Can you work these out from the drawing? Everything is in mm from the part's minimum corner. A direction names the side the tool comes from. Coordinates: 2 decimals unless noted, no trailing zeros. Write each loop counter-clockwise with the first axis right and the second up, starting at its lowest first coordinate (ties: lowest second). Pieces come first, ordered by that corner, then holes. Notation, with made-up numbers: (-7, 39.25) -> (14, 39.25) arc R29 cw to (14, 64.25) -> close; hole circle Ø2 at (82.5, 25). An arc over 180 degrees is marked (long way). Use a Markdown table: item, result. Add a question column.
Item 1: On a 3-axis mill with a long thin cutter (end or side, diameter ignored), from which of +Z, -Z, +X, -X, +Y, -Y can I reach the whole of each face in a straight line? I mean the marked faces 4, 5, 6 and 7. Say none if no direction works.
Item 2: If we mould it in two halves opening along Z, with no side actions, what happens to the marked faces 1, 2 and 3? For each: pulls with the +Z half, pulls with the -Z half, needs draft (parallel to the pull), parting line crosses it, or undercut.
Item 3: Imagine slicing it at A-A, the plane y = 1.5. Write out the boundary of the cut face in (x, z).
Item 4: Will these pins go through, and if not, where does the flat tip stop? pin 1 Ø3.5 at (y, z) = (12, 37.5) entering from +X; pin 2 Ø1.5 at (x, z) = (99.5, 46.5) entering from +Y.
Item 5: Imagine slicing it at B-B, the plane z = 23.5. Write out the boundary of the cut face in (x, y), and give its area (3 significant figures).
Item 6: If I drill on line 1 along X through (y, z) = (2.5, 27.5); line 2 along X through (y, z) = (2.25, 60); line 3 along Y through (x, z) = (103.5, 53.5), over which ranges is the centre line in solid material (lowest first)? Write a range as from..to.
Item 7: Imagine slicing it at C-C, the plane x = 74.5. Write out the boundary of the cut face in (y, z), and give its area (3 significant figures).
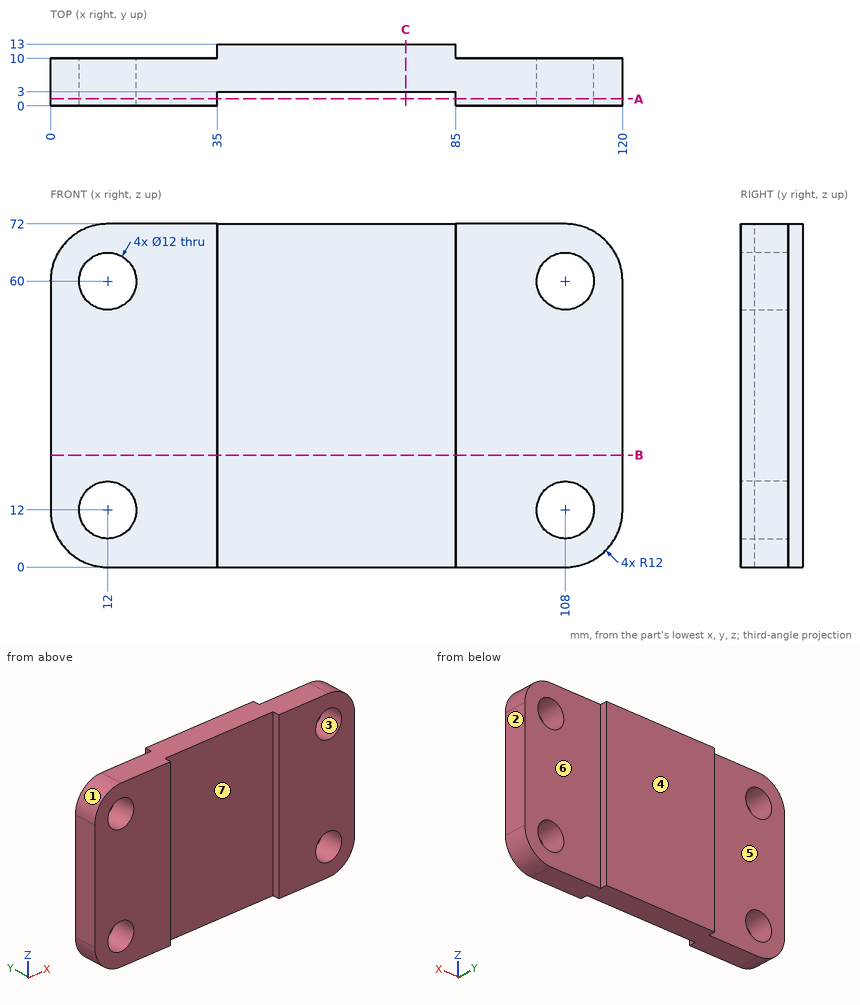
Ans:
| question | item | result |
|---|---|---|
| 1 | face 4 | +Z, -Z, +X, -X, +Y |
| 1 | face 5 | +Z, -Z, -X, +Y |
| 1 | face 6 | +Z, -Z, +X, +Y |
| 1 | face 7 | +Z, -Z, -Y |
| 2 | face 1 | pulls with the +Z half |
| 2 | face 2 | needs draft |
| 2 | face 3 | undercut |
| 3 | outline | (0, 12) arc R12 ccw to (12, 0) -> (35, 0) -> (35, 72) -> (12, 72) arc R12 ccw to (0, 60) -> close; (85, 0) -> (108, 0) arc R12 ccw to (120, 12) -> (120, 60) arc R12 ccw to (108, 72) -> (85, 72) -> close; hole circle Ø12 at (12, 12); hole circle Ø12 at (12, 60); hole circle Ø12 at (108, 12); hole circle Ø12 at (108, 60) |
| 4 | pin 1 | stops at x = 85 |
| 4 | pin 2 | stops at y = 10 |
| 5 | outline | (0, 0) -> (35, 0) -> (35, 3) -> (85, 3) -> (85, 0) -> (120, 0) -> (120, 10) -> (85, 10) -> (85, 13) -> (35, 13) -> (35, 10) -> (0, 10) -> close |
| 5 | area | 1,200 mm^2 |
| 6 | line 1 | x = 0..35, 85..120 |
| 6 | line 2 | x = 0..6, 18..35, 85..102, 114..120 |
| 6 | line 3 | y = 0..10 |
| 7 | outline | (3, 0) -> (13, 0) -> (13, 72) -> (3, 72) -> close |
| 7 | area | 720 mm^2 |
